Design review of the part built by this model. Coordinates are the model's own, in mm. Coordinates: 2 decimals unless noted, no trailing zeros. Loops run counter-clockwise (first coordinate to the right, second up) from the corner with the lowest first, then second, coordinate; pieces in that order, holes last. Notation, with made-up numbers: M 18.5,-17 L 77.5,-17 A20 cw 77.5,4 Z; hole C 1,-36.75 d10. An arc over 180 degrees is marked long. Put each result on its own line as item: value. Start each with the question number.
(1) For probe 1 along Y at (x, z) = (44.25, 0.8); probe 2 along Y at (x, z) = (45, 0.8); probe 3 along X at (y, z) = (44, 2.3), list the stretches that pass through material, from the lowest coordinate up. Write a range as [from, to].
(2) Take a section at A-A, the plane x = 44.25. Give the boundary of the cut face in (y, z).
(3) Take a section at B-B, the plane y = 45.7. Give the boundary of the cut face in (x, z), then the cut area to 3 significant figures.
Autodesk Inventor part; units mm, degrees
ref_plane "YZ Plane" through (0, 0, 0) normal (1, 0, 0) x (0, 1, 0)
ref_plane "XZ Plane" through (0, 0, 0) normal (0, 1, 0) x (-1, 0, 0)
ref_plane "XY Plane" through (0, 0, 0) normal (0, 0, 1) x (1, 0, 0)
sketch "Sketch1" plane through (0, 0, 0) normal (0, 0, 1) x (1, 0, 0)
  line L0 (50.75, 0) -> (50.75, 125.8)
  line L1 (50.75, 125.8) -> (0, 125.8)
  line L2 (0, 125.8) -> (0, 0)
  circle A0 centre (44.25, 10) radius 2.5
  circle A1 centre (44.25, 45.7) radius 2.5
  line L3 (0, 0) -> (50.75, 0)
  dimension "d0" = 50.75
  dimension "d1" = 125.8
  dimension "d2" = 5
  dimension "d3" = 5
  dimension "d14" = 10
  dimension "d15" = 35.7
  dimension "d16" = 6.5
  dimension "d17" = 6.5
extrude "Extrusion1" add sketch "Sketch1" along normal blind 3.1
properties part number "BatteryBracket"
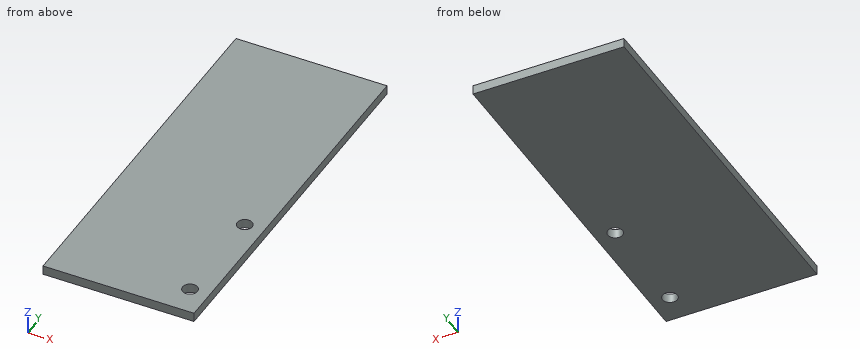
Computed values:
1. probe 1: y = [0, 7.5], [12.5, 43.2], [48.2, 125.8]
1. probe 2: y = [0, 7.62], [12.38, 43.32], [48.08, 125.8]
1. probe 3: x = [0, 42.42], [46.08, 50.75]
2. outline: M 0,0 L 7.5,0 L 7.5,3.1 L 0,3.1 Z; M 12.5,0 L 43.2,0 L 43.2,3.1 L 12.5,3.1 Z; M 48.2,0 L 125.8,0 L 125.8,3.1 L 48.2,3.1 Z
3. outline: M 0,0 L 41.75,0 L 41.75,3.1 L 0,3.1 Z; M 46.75,0 L 50.75,0 L 50.75,3.1 L 46.75,3.1 Z
3. area: 142 mm^2
